from build123d import *

# Parameters (mm, degrees)
SKETCH2_R               = 25
SKETCH2_R_2             = 4.025
SKETCH2_R_3             = 6.25
SKETCH2_R_4             = 2.375
BOSS_EXTRUDE2_DEPTH     = 8
CUT_EXTRUDE1_DEPTH      = 47.637413369
CUT_EXTRUDE1_DEPTH_BACK = 47.637413369
SKETCH3_R               = 2.25
SKETCH2_4_R             = 4.025
CUT_EXTRUDE2_DEPTH      = 4


with BuildPart() as part:
    # Sketch2 → Boss-Extrude2 (new body)
    # profile 1 of 8: a face of its own
    with BuildSketch(Plane.XY):
        with Locations((-3.028012221, -11.407126455)):
            Circle(SKETCH2_R)
        with Locations((-15.028012221, -11.407126455)):
            Circle(SKETCH2_R_2, mode=Mode.SUBTRACT)
        with Locations((-9.028012221, -1.014821609)):
            Circle(SKETCH2_R_2, mode=Mode.SUBTRACT)
        with Locations((2.971987779, -1.014821609)):
            Circle(SKETCH2_R_2, mode=Mode.SUBTRACT)
        with Locations((8.971987779, -11.407126455)):
            Circle(SKETCH2_R_2, mode=Mode.SUBTRACT)
        with Locations((2.971987779, -21.7994313)):
            Circle(SKETCH2_R_2, mode=Mode.SUBTRACT)
        with Locations((-9.028012221, -21.7994313)):
            Circle(SKETCH2_R_2, mode=Mode.SUBTRACT)
        with Locations((-3.028012221, -11.407126455)):
            Circle(SKETCH2_R_3, mode=Mode.SUBTRACT)
    # profile 2 of 8: a face of its own
    with BuildSketch(Plane.XY):
        with Locations((-15.028012221, -11.407126455)):
            Circle(SKETCH2_R_2)
        with Locations((-15.028012221, -11.407126455)):
            Circle(SKETCH2_R_4, mode=Mode.SUBTRACT)
    # profile 3 of 8: a face of its own
    with BuildSketch(Plane.XY):
        with Locations((-3.028012221, -11.407126455)):
            Circle(SKETCH2_R_3)
    # profile 4 of 8: a face of its own
    with BuildSketch(Plane.XY):
        with Locations((-9.028012221, -1.014821609)):
            Circle(SKETCH2_R_2)
        with Locations((-9.028012221, -1.014821609)):
            Circle(SKETCH2_R_4, mode=Mode.SUBTRACT)
    # profile 5 of 8: a face of its own
    with BuildSketch(Plane.XY):
        with Locations((2.971987779, -1.014821609)):
            Circle(SKETCH2_R_2)
        with Locations((2.971987779, -1.014821609)):
            Circle(SKETCH2_R_4, mode=Mode.SUBTRACT)
    # profile 6 of 8: a face of its own
    with BuildSketch(Plane.XY):
        with Locations((8.971987779, -11.407126455)):
            Circle(SKETCH2_R_2)
        with Locations((8.971987779, -11.407126455)):
            Circle(SKETCH2_R_4, mode=Mode.SUBTRACT)
    # profile 7 of 8: a face of its own
    with BuildSketch(Plane.XY):
        with Locations((2.971987779, -21.7994313)):
            Circle(SKETCH2_R_2)
        with Locations((2.971987779, -21.7994313)):
            Circle(SKETCH2_R_4, mode=Mode.SUBTRACT)
    # profile 8 of 8: a face of its own
    with BuildSketch(Plane.XY):
        with Locations((-9.028012221, -21.7994313)):
            Circle(SKETCH2_R_2)
        with Locations((-9.028012221, -21.7994313)):
            Circle(SKETCH2_R_4, mode=Mode.SUBTRACT)
    extrude(amount=BOSS_EXTRUDE2_DEPTH)

    # Sketch3 → Cut-Extrude1 (cut, two sides: drawn at the far end of the back side and taken through both)
    with BuildSketch(Plane(origin=(0, 0, 0), x_dir=(-1, 0, 0), z_dir=(0, 0, -1)).offset(-CUT_EXTRUDE1_DEPTH_BACK)):
        with Locations((-9.471987779, 2.592873545)):
            Circle(SKETCH3_R)
        with Locations((15.528012221, 2.592873545)):
            Circle(SKETCH3_R)
        with Locations((15.528012221, -25.407126455)):
            Circle(SKETCH3_R)
        with Locations((-9.471987779, -25.407126455)):
            Circle(SKETCH3_R)
    extrude(amount=CUT_EXTRUDE1_DEPTH + CUT_EXTRUDE1_DEPTH_BACK, mode=Mode.SUBTRACT)

    # Sketch2<4> → Cut-Extrude2 (cut)
    with BuildSketch(Plane.XY):
        with Locations((-15.028012221, -11.407126455)):
            Circle(SKETCH2_4_R)
        with Locations((-9.028012221, -1.014821609)):
            Circle(SKETCH2_4_R)
        with Locations((2.971987779, -1.014821609)):
            Circle(SKETCH2_4_R)
        with Locations((8.971987779, -11.407126455)):
            Circle(SKETCH2_4_R)
        with Locations((2.971987779, -21.7994313)):
            Circle(SKETCH2_4_R)
        with Locations((-9.028012221, -21.7994313)):
            Circle(SKETCH2_4_R)
    extrude(amount=CUT_EXTRUDE2_DEPTH, mode=Mode.SUBTRACT)


solid = part.part
The model under review builds one solid part; all positions refer to its coordinate system, in mm. A direction names the side the tool comes from. Give positions to 0.01 mm unless a question says otherwise; leave off trailing zeros. Order: outer loops, then holes, each group sorted by start corner. A loop starts at its lowest first (then second) coordinate and runs counter-clockwise, first axis right, second up. Notation, with made-up numbers: (-36, 41) -> (11, 41) arc R18 cw to (11, 76) -> close; hole circle Ø11 at (-13, 85). An arc over 180 degrees is marked (long way). Write item = value, one per line. Start each with the question number.
(1) Tool access review of faces 1 (the cylindrical face through (-6.834, -1.924, 5.972)), 2 (the flat face through (5, -3, 4)): name each direction out of +Z, -Z, +X, -X, +Y, -Y from which nothing blocks a thin tool from reaching the whole face with its end or side.
(2) Take a section at C-C (z = 2). State how many separate pieces and enclosed holes the cut face has, plus the area to 3 significant figures.
(3) For pin 1 Ø5.5 at (x, y) = (-9.03, -21.8) entering from -Z; pin 2 Ø1.5 at (y, z) = (-3.5, 4.5) entering from -X; pin 3 Ø3 at (x, y) = (-15.03, -11.41) entering from +Z; pin 4 Ø9.5 at (x, y) = (8.97, -11.41) entering from -Z, all flat-tipped, find the tip position at first contact; note any pin that passes through.
(4) Take a section at B-B (x = 4). Write out the cut boundary in (y, z), plus the area to 3 significant figures.
(5) Take a section at D-D (x = 10.5). Write out the cut boundary in (y, z).
(6) For L1, parallel to Y at x = 1.5, z = 1; L2, parallel to X at y = -25, z = 7.5; L3, parallel to Y at x = 2, z = 3, list the stretches that pass through material, from the lowest coordinate up. Write a range as from..to.
(7) Take a section at A-A (y = -10). Write out the cut boundary in (x, z).
(8) Draft analysis for pull direction Y (two halves, no side actions). For faces 3 (the cylindrical face through (-12.834, -12.317, 5.972)), 4 (the cylindrical face through (-8.448, -35.813, 3.944)), 5 (the flat face through (-3, -11, 8)), state which applies: +Y half, -Y half, draft (parallel to the pull), parting line (faces both ways), or undercut.
Returned:
q1.face_1 = +Z, -Z
q1.face_2 = -Z
q2.separate_pieces = 1
q2.enclosed_holes = 10
q2.area = 1,590 mm²
q3.pin_1 = 4
q3.pin_2 = -26.98
q3.pin_3 = through
q3.pin_4 = 0
q4.outline = (-35.4, 0) -> (-25.69, 0) -> (-25.69, 4) -> (-23.94, 4) -> (-23.94, 8) -> (-35.4, 8) -> close; (-19.66, 4) -> (-17.91, 4) -> (-17.91, 0) -> (-4.91, 0) -> (-4.91, 4) -> (-3.16, 4) -> (-3.16, 8) -> (-19.66, 8) -> close; (1.13, 4) -> (2.88, 4) -> (2.88, 0) -> (12.58, 0) -> (12.58, 8) -> (1.13, 8) -> close
q4.area = 287 mm²
q5.outline = (-32.43, 0) -> (-27.41, 0) -> (-27.41, 8) -> (-32.43, 8) -> close; (-23.41, 0) -> (-15.13, 0) -> (-15.13, 4) -> (-13.23, 4) -> (-13.23, 8) -> (-23.41, 8) -> close; (-9.59, 4) -> (-7.68, 4) -> (-7.68, 0) -> (0.59, 0) -> (0.59, 8) -> (-9.59, 8) -> close; (4.59, 0) -> (9.62, 0) -> (9.62, 8) -> (4.59, 8) -> close
q6.L1 = -35.99..-25.55, -18.05..-4.76, 2.73..13.18
q6.L2 = -24.01..-17.74, -13.32..7.26, 11.68..17.95
q6.L3 = -35.9..-25.71, -17.89..-4.92, 2.89..13.08
q7.outline = (-27.99, 0) -> (-18.8, 0) -> (-18.8, 4) -> (-16.94, 4) -> (-16.94, 8) -> (-27.99, 8) -> close; (-13.11, 4) -> (-11.26, 4) -> (-11.26, 0) -> (5.2, 0) -> (5.2, 4) -> (7.06, 4) -> (7.06, 8) -> (-13.11, 8) -> close; (10.89, 4) -> (12.74, 4) -> (12.74, 0) -> (21.93, 0) -> (21.93, 8) -> (10.89, 8) -> close
q8.face_3 = undercut
q8.face_4 = parting line
q8.face_5 = draft
